Geometry check sheet. Reference: the model listing, model coordinates, mm. Face numbers are marked on the shaded views. A direction names the side the tool comes from. Give positions to 0.01 mm unless a question says otherwise; leave off trailing zeros. Order: outer loops, then holes, each group sorted by start corner. A loop starts at its lowest first (then second) coordinate and runs counter-clockwise, first axis right, second up. Notation, with made-up numbers: M 21,16.5 L 27,16.5 A33 cw 27,46.5 Z; hole C 26,48 d2. An arc over 180 degrees is marked long. Put each result on its own line as item: value. Start each with the question number.
Q1. Access from +Z, -Z, +X, -X, +Y, -Y to the whole of each face (thin tool, end or side, straight path). Record for the marked faces 4 and 5.
Q2. Section check B-B on z = 2.15. Record the cut outline in (x, y).
Q3. Section check A-A on y = 6.5. Record the cut outline in (x, z), then the cut area to 3 significant figures.
Q4. Go/stop test with flat-tipped pins: pin 1 (1.3 mm diameter, centred on x = 14.5, z = 2, fed in from +Y); pin 2 (11 mm diameter, centred on x = 3, y = -2.5, fed in from +Z); pin 3 (0.6 mm diameter, centred on x = 15, z = 1.5, fed in from -Y). Record where each tip stops, or that it passes through.
Q5. Mould release check, pull along X, two halves, no side actions. Record for the marked faces 1, 2 and 3: +X half, -X half, draft (parallel to the pull), parting line (faces both ways), or undercut.
Q6. Material ranges on L1, parallel to X at y = 5.5, z = 1.1; L2, parallel to Y at x = -11.5, z = 0.6; L3, parallel to X at y = 3, z = 0.9, recorded low to high.
Autodesk Inventor part; units mm, degrees
ref_plane "YZ Plane" through (0, 0, 0) normal (1, 0, 0) x (0, 1, 0)
ref_plane "XZ Plane" through (0, 0, 0) normal (0, 1, 0) x (-1, 0, 0)
ref_plane "XY Plane" through (0, 0, 0) normal (0, 0, 1) x (1, 0, 0)
sketch "Sketch1" plane through (0, 0, 0) normal (0, 0, 1) x (1, 0, 0)
  line L0 (-20.3, 12) -> (15.5, 12)
  line L1 (15.5, 12) -> (15.5, -12)
  line L2 (15.5, -12) -> (-20.3, -12)
  line L3 (-20.3, -12) -> (-20.3, 12)
  line L4 (-14.3, 8.8) -> (14.3, 8.8)
  line L5 (14.3, 8.8) -> (14.3, -8.8)
  line L6 (14.3, -8.8) -> (-14.3, -8.8)
  line L7 (-14.3, -8.8) -> (-14.3, 8.8)
  line L8 (-8, 5) -> (8, 5)
  line L9 (8, 5) -> (8, -5)
  line L10 (8, -5) -> (-8, -5)
  line L11 (-8, -5) -> (-8, 5)
  point P0 (0, 0)
  point P1 (14.3, 0)
  point P2 (0, 8.8)
  point P3 (15.5, 0)
  point P4 (8, 0)
  point P5 (0, 5)
  dimension "d0" = 28.6
  dimension "d1" = 17.6
  dimension "d2" = 1.2
  dimension "d3" = 6
  dimension "d4" = 24
  dimension "d9" = 10
  dimension "d10" = 16
extrude "Extrusion1" add sketch "Sketch1" against normal blind 2 contours L0 L1 L2 L3 | L4 L5 L6 L7 | L8 L9 L10 L11
extrude "Extrusion2" add sketch "Sketch1" along normal blind 3 contours L0 L1 L2 L3
extrude "Extrusion3" add sketch "Sketch1" along normal blind 1 contours L8 L9 L10 L11
fillet "Fillet1" radius 2 4 edges at (-20.3, -12, 0.5) (-20.3, 12, 0.5) (15.5, 12, 0.5) (15.5, -12, 0.5)
fillet "Fillet2" radius 0.5 8 edges at (14.3, 8.8, 1.5) (14.3, -8.8, 1.5) (-14.3, 8.8, 1.5) (-14.3, -8.8, 1.5) (-8, 5, 0.5) (-8, -5, 0.5) (8, -5, 0.5) (8, 5, 0.5)
sketch "Sketch2" plane through (15.5, -10, -2) normal (1, 0, 0) x (0, 0, -1)
  line L0 (-5, 0) -> (-5, 20)
  line L1 (-5, 5) -> (-3, 5)
  line L2 (-3, 5) -> (-3, 15)
  line L3 (-3, 15) -> (-5, 15)
  line L4 (-5, 15) -> (-5, 5)
  point P0 (-2, 10)
  point P1 (-3, 10)
  dimension "d21" = 10
  dimension "d22" = 2
extrude "Extrusion4" cut sketch "Sketch2" against normal up to surface (1.2 mm away)
chamfer "Chamfer3" distance 0.3 angle 45 4 edges at (14.9, -5, 1) (14.9, -5, 3) (14.9, 5, 1) (14.9, 5, 3)
chamfer "Chamfer1" distance 1 angle 45 8 edges at (-8, 0, 0) (-7.8536, 4.8536, 0) (0, 5, 0) (7.8536, 4.8536, 0) (8, 0, 0) (7.8536, -4.8536, 0) (0, -5, 0) (-7.8536, -4.8536, 0)
chamfer "Chamfer2" distance 0.4 angle 45 34 edges at (0, 8.8, 0) (-14.1536, 8.6536, 0) (-14.3, 0, 0) (-14.1536, -8.6536, 0) (0, -8.8, 0) (14.1536, -8.6536, 0) (14.3, 0, 0) (14.1536, 8.6536, 0) (0, 8.8, 3) (14.1536, 8.6536, 3) (14.3, -6.8, 3) (14.3, 6.8, 3) (14.1536, -8.6536, 3) (0, -8.8, 3) (-14.1536, -8.6536, 3) (-14.3, 0, 3) (-14.1536, 8.6536, 3) (-2.4, 12, 3) (-19.7142, 11.4142, 3) (-20.3, 0, 3) (-19.7142, -11.4142, 3) (-2.4, -12, 3) (14.9142, -11.4142, 3) (15.5, -7.65, 3) (15.5, 7.65, 3) (14.9142, 11.4142, 3) (-20.3, 0, -2) (-19.7142, 11.4142, -2) (-2.4, 12, -2) (14.9142, 11.4142, -2) (15.5, 0, -2) (14.9142, -11.4142, -2) (-2.4, -12, -2) (-19.7142, -11.4142, -2)
properties part number "tp4056-pad" material "ABS Plastic"
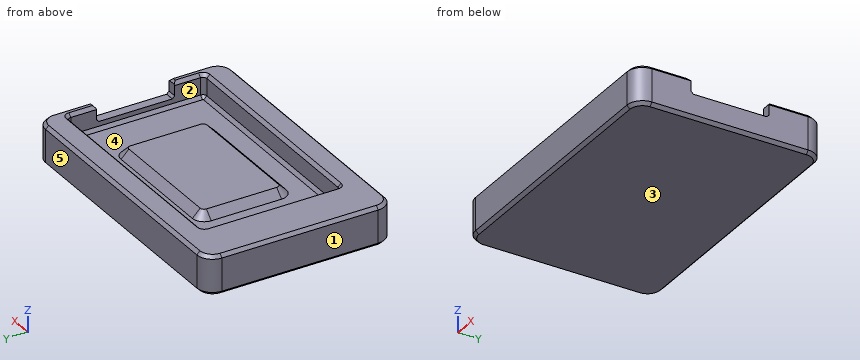
Results found:
1. face 4: +Z
1. face 5: +Z, -Z, +X, -X, +Y
2. outline: M -20.3,-10 A2 ccw -18.3,-12 L 13.5,-12 A2 ccw 15.5,-10 L 15.5,-5 L 14.3,-5 L 14.3,-8.3 A0.5 cw 13.8,-8.8 L -13.8,-8.8 A0.5 cw -14.3,-8.3 L -14.3,8.3 A0.5 cw -13.8,8.8 L 13.8,8.8 A0.5 cw 14.3,8.3 L 14.3,5 L 15.5,5 L 15.5,10 A2 ccw 13.5,12 L -18.3,12 A2 ccw -20.3,10 Z
3. outline: M -20.3,-1.6 L -19.9,-2 L 15.1,-2 L 15.5,-1.6 L 15.5,2.6 L 15.1,3 L 14.7,3 L 14.3,2.6 L 14.3,0.4 L 13.9,0 L -13.9,0 L -14.3,0.4 L -14.3,2.6 L -14.7,3 L -19.9,3 L -20.3,2.6 Z
3. area: 92.9 mm^2
4. pin 1: stops at y = 11.97
4. pin 2: stops at z = 1
4. pin 3: stops at y = -11.6
5. face 1: -X half
5. face 2: undercut
5. face 3: draft
6. L1: x = -20.3 to -14.3, 14.3 to 15.5
6. L2: y = -12 to -8.8, 8.8 to 12
6. L3: x = -20.3 to -14.3, -8.1 to 8.1, 14.3 to 15.5
